For this review, take the finished solid that the model builds, in its own axes (mm). A direction names the side the tool comes from. Coordinates: 2 decimals unless noted, no trailing zeros. Order: outer loops, then holes, each group sorted by start corner. A loop starts at its lowest first (then second) coordinate and runs counter-clockwise, first axis right, second up. Notation, with made-up numbers: (6.25, 49.5) -> (31.25, 49.5) arc R21 ccw to (31.25, 62.5) -> close; hole circle Ø5 at (17.5, 73.25). An arc over 180 degrees is marked (long way). Return JSON: item names as keys, results as strings. Group by question number.
Item 1: Insertion check: pin 1 (3 mm diameter, centred on y = 332.5, z = 4.5, fed in from -X); pin 2 (1 mm diameter, centred on y = 227.5, z = 4.5, fed in from -X). Each pin has a flat end and moves straight along its axis. Give the tip position at first contact, or say it passes through.
Item 2: For line 1 along X through (y, z) = (467.5, 0.5); line 2 along Y through (x, z) = (7, 1.5); line 3 along Z through (x, y) = (5.25, 416.5), list the stretches that pass through material, from the lowest coordinate up.
Item 3: Machinability: for faces 1 (the cylindrical face through (-6, 34, 0)), 2 (the flat face through (0, 0, 0)), 3 (the flat face through (5.2, 489, -0.1)), which of the approach directions +Z, -Z, +X, -X, +Y, -Y give a long, thin tool a straight path to every point of the face, cutting with its end or side? Answer none if there is none.
Item 4: Take a section at A-A (z = 0). Write out the cut boundary in (x, y), then the cut area to 3 significant figures.
Item 5: Take a section at C-C (y = 414.5). Write out the cut boundary in (x, z), then the cut area to 3 significant figures.
Item 6: Take a section at B-B (x = 0). Write out the cut boundary in (y, z).
```python
from build123d import *

# Parameters (mm, degrees)
SKETCH_R     = 5
PAD_DEPTH    = 15
SKETCH001_R  = 6
PAD001_DEPTH = 39
SKETCH002_R  = 8
PAD002_DEPTH = 435
SKETCH003_R  = 5
PAD003_DEPTH = 11


with BuildPart() as part:
    # Sketch → Pad (new body)
    with BuildSketch(Plane.XZ):
        Circle(SKETCH_R)
    extrude(amount=-PAD_DEPTH)

    # Sketch001 (on Face3 of Pad) → Pad001 (join)
    with BuildSketch(Plane(origin=(0, 15, 0), x_dir=(1, 0, 0), z_dir=(0, 1, 0))):
        Circle(SKETCH001_R)
    extrude(amount=PAD001_DEPTH)

    # Sketch002 (on Face3 of Pad001) → Pad002 (join)
    with BuildSketch(Plane(origin=(0, 54, 0), x_dir=(1, 0, 0), z_dir=(0, 1, 0))):
        Circle(SKETCH002_R)
    extrude(amount=PAD002_DEPTH)

    # Sketch003 (on Face3 of Pad002) → Pad003 (join)
    with BuildSketch(Plane(origin=(0, 489, 0), x_dir=(1, 0, 0), z_dir=(0, 1, 0))):
        Circle(SKETCH003_R)
    extrude(amount=PAD003_DEPTH)


solid = part.part
```
Findings below:
{
 "1": {"pin 1": "stops at x = -7.42", "pin 2": "stops at x = -6.93"},
 "2": {"line 1": "x = -7.98 to 7.98", "line 2": "y = 54 to 489", "line 3": "z = -6.04 to 6.04"},
 "3": {"face 1": "-Y", "face 2": "+Z, -Z, +X, -X, -Y", "face 3": "+Y"},
 "4": {"outline": "(-8, 54) -> (-6, 54) -> (-6, 15) -> (-5, 15) -> (-5, 0) -> (5, 0) -> (5, 15) -> (6, 15) -> (6, 54) -> (8, 54) -> (8, 489) -> (5, 489) -> (5, 500) -> (-5, 500) -> (-5, 489) -> (-8, 489) -> close", "area": "7,690 mm2"},
 "5": {"outline": "circle Ø16 at (0, 0)", "area": "201 mm2"},
 "6": {"outline": "(0, -5) -> (15, -5) -> (15, -6) -> (54, -6) -> (54, -8) -> (489, -8) -> (489, -5) -> (500, -5) -> (500, 5) -> (489, 5) -> (489, 8) -> (54, 8) -> (54, 6) -> (15, 6) -> (15, 5) -> (0, 5) -> close"}
}
